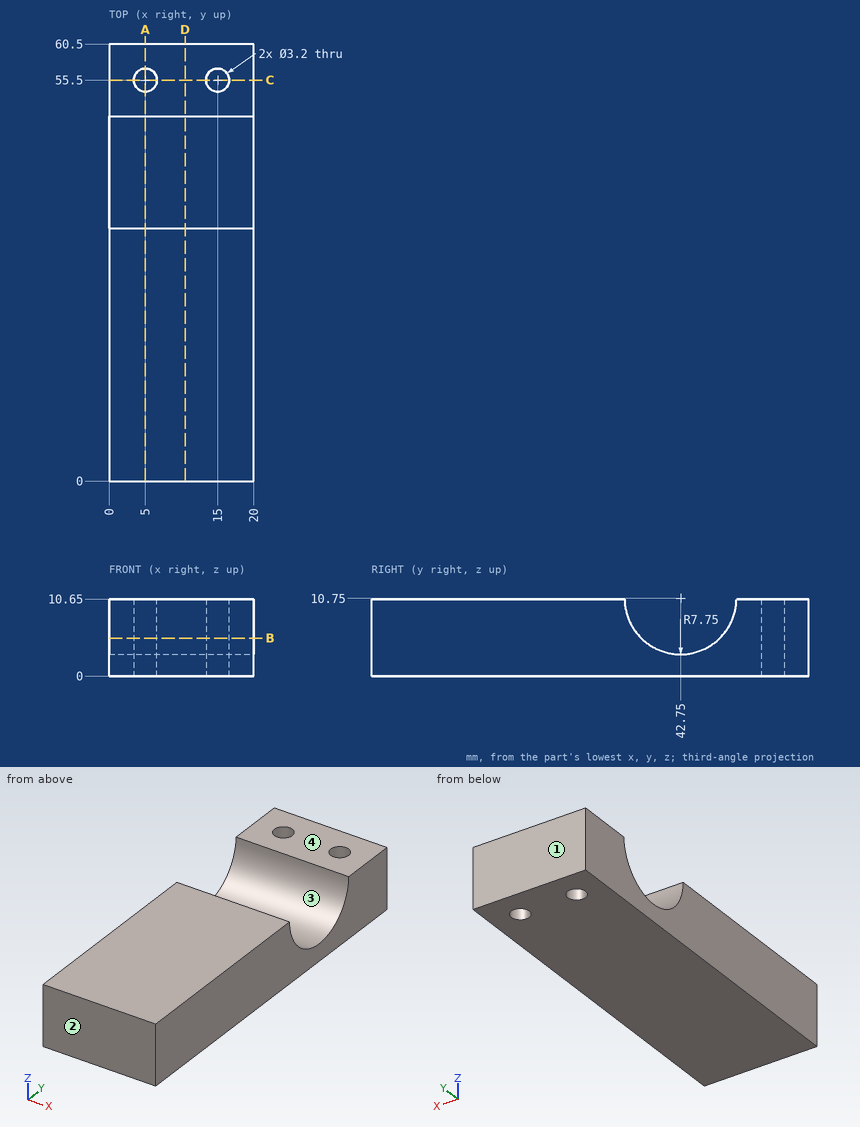
The figure shows three views and two pictorial views of one solid part (mm, origin at its lowest corner). Answer the questions. Give positions to 0.01 mm unless a question says otherwise; leave off trailing zeros. Loops run counter-clockwise (first coordinate to the right, second up) from the corner with the lowest first, then second, coordinate; pieces in that order, holes last. Notation, with made-up numbers: M 37.25,70.25 L 90.25,70.25 A19 cw 90.25,89.25 Z; hole C 12.25,60 d1. An arc over 180 degrees is marked long. Write each question's results on one line, items separated by ' | '.
1. Section B-B on z = 5.25 is taken. Give the vertices of the cut face in (x, y).
Values:
outline: M 0,0 L 20,0 L 20,37.29 L 0,37.29 Z; M 0,48.21 L 20,48.21 L 20,60.5 L 0,60.5 Z; hole C 5,55.5 d3.2; hole C 15,55.5 d3.2
2. Straight lines are drawn through the part: line 1 (X direction, y = 55.5, z = 4); line 2 (Y direction, x = 5.5, z = 5); line 3 (Y direction, x = 5, z = 6.25). For each, find the intervals that lie inside material, in ascending order. Write a range as [from, to].
Values:
line 1: x = [0, 3.4], [6.6, 13.4], [16.6, 20] | line 2: y = [0, 37.55], [47.95, 53.98], [57.02, 60.5] | line 3: y = [0, 36.44], [49.06, 53.9], [57.1, 60.5]
3. The mould has two halves that part along Y. Classify the marked faces 1, 2, 3 and 4: pulls with the +Y half, pulls with the -Y half, needs draft (parallel to the pull), parting line crosses it, or undercut.
Values:
face 1: pulls with the +Y half | face 2: pulls with the -Y half | face 3: undercut | face 4: needs draft
4. Given pin 1 (4 mm diameter, centred on x = 15, y = 55.5, fed in from +Z); pin 2 (3 mm diameter, centred on x = 10.5, y = 46, fed in from +Z), each flat-ended and moving along its own axis, determine where each tip first touches the part or whether it passes through.
Values:
pin 1: stops at z = 10.65 | pin 2: stops at z = 4.63
5. Section C-C on y = 55.5 is taken. Give the vertices of the cut face in (x, z).
Values:
outline: M 0,0 L 3.4,0 L 3.4,10.65 L 0,10.65 Z; M 6.6,0 L 13.4,0 L 13.4,10.65 L 6.6,10.65 Z; M 16.6,0 L 20,0 L 20,10.65 L 16.6,10.65 Z
6. Section A-A on x = 5 is taken. Give the vertices of the cut face in (y, z), plus the area to 3 significant figures.
Values:
outline: M 0,0 L 53.9,0 L 53.9,10.65 L 50.5,10.65 A7.75 cw 35,10.65 L 0,10.65 Z; M 57.1,0 L 60.5,0 L 60.5,10.65 L 57.1,10.65 Z | area: 517 mm^2
7. Section D-D on x = 10.5 is taken. Give the vertices of the cut face in (y, z), plus the area to 3 significant figures.
Values:
outline: M 0,0 L 60.5,0 L 60.5,10.65 L 50.5,10.65 A7.75 cw 35,10.65 L 0,10.65 Z | area: 552 mm^2
